```python
from build123d import *

# Parameters (mm, degrees)
F0_R     = 139.7
F0_R_2   = 11.1125
F0_R_3   = 76.2
F1_DEPTH = 23.876
F2_R     = 95.25
F2_R_2   = 76.2
F3_DEPTH = 3.175
F4_R     = 2.54


with BuildPart() as f1:
    # F0 (on Front) → F1 (new body)
    with BuildSketch(Plane.XZ):
        Circle(F0_R)
        with Locations((-85.312433, -85.312433)):
            Circle(F0_R_2, mode=Mode.SUBTRACT)
        with Locations((0, -120.65)):
            Circle(F0_R_2, mode=Mode.SUBTRACT)
        with Locations((85.312433, -85.312433)):
            Circle(F0_R_2, mode=Mode.SUBTRACT)
        with Locations((-120.65, 0)):
            Circle(F0_R_2, mode=Mode.SUBTRACT)
        with Locations((-85.312433, 85.312433)):
            Circle(F0_R_2, mode=Mode.SUBTRACT)
        Circle(F0_R_3, mode=Mode.SUBTRACT)
        with Locations((120.65, 0)):
            Circle(F0_R_2, mode=Mode.SUBTRACT)
        with Locations((0, 120.65)):
            Circle(F0_R_2, mode=Mode.SUBTRACT)
        with Locations((85.312433, 85.312433)):
            Circle(F0_R_2, mode=Mode.SUBTRACT)
    extrude(amount=F1_DEPTH)

    # F2 (on face) → F3 (join)
    with BuildSketch(Plane.XZ.offset(23.876)):
        Circle(F2_R)
        Circle(F2_R_2, mode=Mode.SUBTRACT)
    extrude(amount=F3_DEPTH)

    # F4
    f4_edges = [f1.edges().sort_by_distance(p)[0] for p in [
        (-139.7, -23.876, 0),
        (-139.7, 0, 0),
    ]]
    fillet(f4_edges, radius=F4_R)


solid = f1.part
```
For this review, take the finished solid that the model builds, in its own axes (mm). A direction names the side the tool comes from. Coordinates: 2 decimals unless noted, no trailing zeros. Write each loop counter-clockwise with the first axis right and the second up, starting at its lowest first coordinate (ties: lowest second). Pieces come first, ordered by that corner, then holes. Notation, with made-up numbers: (-14.5, -6) - (16.5, -6) arc R17 cw to (16.5, 27) - close; hole circle Ø3 at (36, 37). An arc over 180 degrees is marked (long way). Put each result on its own line as item: value.
1. Add section A-A, the plane z = 0. Give the boundary of the cut face in (x, y).
Values found:
outline: (-139.7, -21.34) arc R2.54 ccw to (-137.16, -23.88) - (-131.76, -23.88) - (-131.76, 0) - (-137.16, 0) arc R2.54 ccw to (-139.7, -2.54) - close; (-109.54, -23.88) - (-95.25, -23.88) - (-95.25, -27.05) - (-76.2, -27.05) - (-76.2, 0) - (-109.54, 0) - close; (76.2, -27.05) - (95.25, -27.05) - (95.25, -23.88) - (109.54, -23.88) - (109.54, 0) - (76.2, 0) - close; (131.76, -23.88) - (137.16, -23.88) arc R2.54 ccw to (139.7, -21.34) - (139.7, -2.54) arc R2.54 ccw to (137.16, 0) - (131.76, 0) - close
2. Mouldability with a two-part tool opening along X and no side actions: class faces 1 (the flat face through (-43, -27.051, 64)), 2 (the cylindrical face through (109.55, -11.77, 0.49)), 3 (the cylindrical face through (-110.86, -11.81, -85.01)) as released by +X, released by -X, zero draft, split by the parting line, or undercut.
Values found:
face 1: zero draft
face 2: undercut
face 3: split by the parting line
3. Add section C-C, the plane y = -16. Count the separate pieces of the cut face and the enclosed holes in it, then the cut area to 3 significant figures.
Values found:
separate pieces: 1
enclosed holes: 9
area: 40,000 mm²
4. Wall thickness on probe 1 along Z at (x, y) = (0, -14); probe 2 along Z at (x, y) = (3.5, -18); probe 3 along Z at (x, y) = (94.5, -5): over which ranges is each line inside the solid? List them lowest first.
Values found:
probe 1: -139.7 to -131.76, -109.54 to -76.2, 76.2 to 109.54, 131.76 to 139.7
probe 2: -139.66 to -131.2, -110.1 to -76.12, 76.12 to 110.1, 131.2 to 139.66
probe 3: -102.89 to -91.56, -79.06 to 79.06, 91.56 to 102.89
5. Add section B-B, the plane x = 0. Give the boundary of the cut face in (y, z), then the cut area to 3 significant figures.
Values found:
outline: (-27.05, -95.25) - (-23.88, -95.25) - (-23.88, -109.54) - (0, -109.54) - (0, -76.2) - (-27.05, -76.2) - close; (-27.05, 76.2) - (0, 76.2) - (0, 109.54) - (-23.88, 109.54) - (-23.88, 95.25) - (-27.05, 95.25) - close; (-23.88, -137.16) arc R2.54 ccw to (-21.34, -139.7) - (-2.54, -139.7) arc R2.54 ccw to (0, -137.16) - (0, -131.76) - (-23.88, -131.76) - close; (-23.88, 131.76) - (0, 131.76) - (0, 137.16) arc R2.54 ccw to (-2.54, 139.7) - (-21.34, 139.7) arc R2.54 ccw to (-23.88, 137.16) - close
area: 2,090 mm²
6. Machinability: for faces 4 (the cylindrical face through (-75.587, -25.441, -57.958)), 5 (the cylindrical face through (-80.185, -11.771, 75.454)), which of the approach directions +Z, -Z, +X, -X, +Y, -Y give a long, thin tool a straight path to every point of the face, cutting with its end or side? Answer none if there is none.
Values found:
face 4: -Y
face 5: +Y, -Y
7. For pin 1 (10 mm diameter, centred on y = -9, z = 47, fed in from -X); pin 2 (6 mm diameter, centred on x = -105.5, z = 89, fed in from +Y); pin 3 (10 mm diameter, centred on y = -13, z = 56, fed in from -X); pin 4 (5 mm diameter, centred on y = -22.5, z = 103, fed in from -X), all flat-tipped, find the tip position at first contact; note any pin that passes through.
Values found:
pin 1: x = -133.24
pin 2: y = 0
pin 3: x = -130.06
pin 4: x = -96.87
